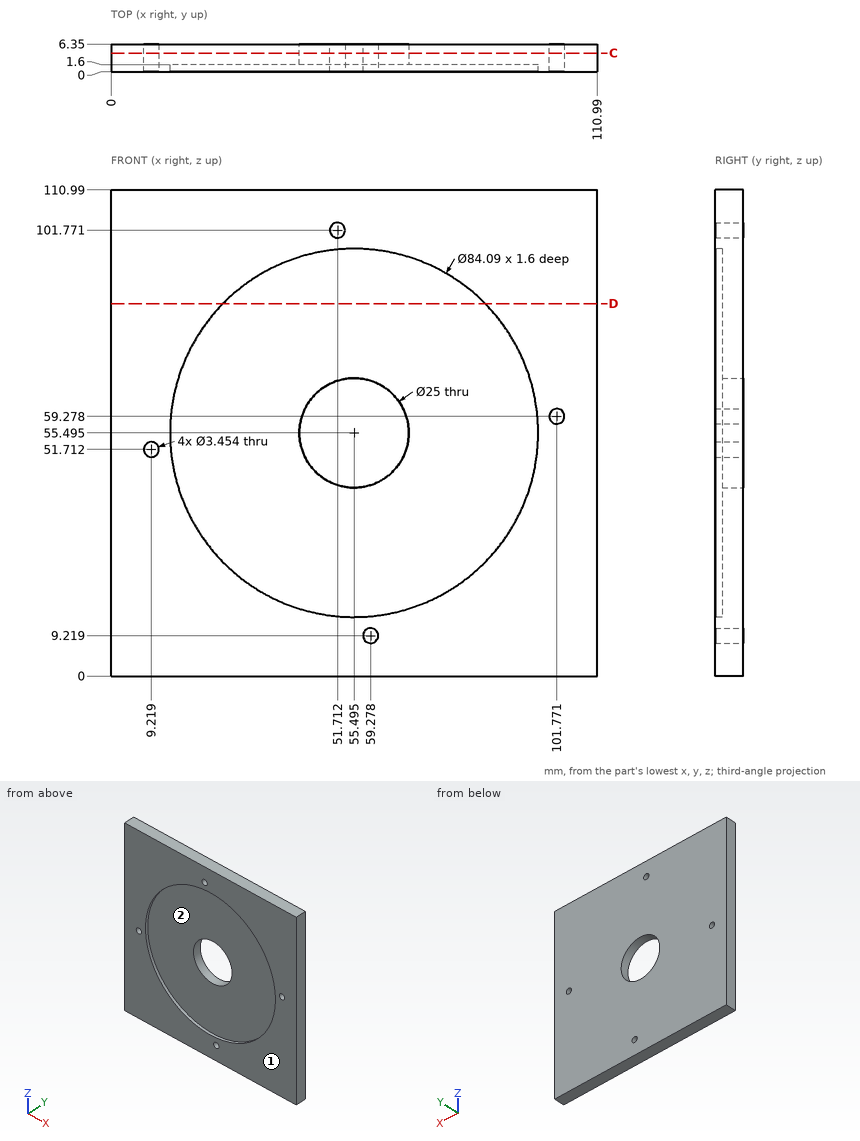
Check sheet for the drawn part. Datum: minimum x, y, z corner. Units: mm. Round coordinates to 2 decimals unless told otherwise and drop trailing zeros. Order: outer loops, then holes, each group sorted by start corner. A loop starts at its lowest first (then second) coordinate and runs counter-clockwise, first axis right, second up.
1. Go/stop test with a flat-tipped pin: P1, Ø6, axis at x = 57.5, z = 17.5, coming from the -Y side. Record where the tip stops, or that it passes through.
Final values:
P1: stops at y = 1.6
2. Section check C-C on y = 4.25. Record the cut outline in (x, z) (1 decimal), then the cut area to 3 significant figures.
Final values:
outline: (0, 0) - (111, 0) - (111, 111) - (0, 111) - close; hole circle Ø3.5 at (9.2, 51.7); hole circle Ø25 at (55.5, 55.5); hole circle Ø3.5 at (51.7, 101.8); hole circle Ø3.5 at (59.3, 9.2); hole circle Ø3.5 at (101.8, 59.3)
area: 11,800 mm2
3. Release check for a two-part mould opening along X. For the marked faces 1 and 2 record: +X half, -X half, draft (parallel to the pull), parting line (faces both ways), or undercut.
Final values:
face 1: draft
face 2: undercut
4. Thickness scan on L1, parallel to Z at x = 53, y = 5.75 (1 decimal); L2, parallel to Y at x = 38, z = 18.5; L3, parallel to Z at x = 55, y = 2.25 (1 decimal). Record the ranges inside material, lowest first.
Final values:
L1: z = 0 to 43.2, 67.7 to 100.6, 102.9 to 111
L2: y = 1.6 to 6.35
L3: z = 0 to 43, 68 to 111
5. Section check D-D on z = 85. Record the cut outline in (x, y), then the cut area to 3 significant figures.
Final values:
outline: (0, 0) - (25.54, 0) - (25.54, 1.6) - (85.45, 1.6) - (85.45, 0) - (110.99, 0) - (110.99, 6.35) - (0, 6.35) - close
area: 609 mm2
